Source: CAD feature listing. Evaluate the final solid. Frame: model axes, mm. A direction names the side the tool comes from. Round coordinates to 2 decimals unless told otherwise and drop trailing zeros. Write each loop counter-clockwise with the first axis right and the second up, starting at its lowest first coordinate (ties: lowest second). Pieces come first, ordered by that corner, then holes.
from build123d import *

# Parameters (mm, degrees)
F0_W     = 25.4
F0_H     = 25.4
F0_W_2   = 19.05
F0_H_2   = 19.05
F1_DEPTH = 1244.6


with BuildPart() as f1:
    # F0 (on Right) → F1 (new body)
    with BuildSketch(Plane.YZ):
        with Locations((12.7, 12.7)):
            Rectangle(F0_W, F0_H)
        with Locations((12.7, 12.7)):
            Rectangle(F0_W_2, F0_H_2, mode=Mode.SUBTRACT)
    extrude(amount=-F1_DEPTH)


solid = f1.part
1) Pull-direction query (Z, two-part tool) for faces 1 (the face through (-614, 13, 25.4)), 2 (the face through (-1244.6, 24, 13)), 3 (the face through (-614, 13, 22.225)); classes: released by +Z, released by -Z, zero draft, split by the parting line, or undercut.
Taken from the geometry:
face 1: released by +Z
face 2: zero draft
face 3: undercut
2) Contact query for a flat-ended pin moving along its axis: P1, Ø2, axis at x = -709.5, z = 21, coming from the -Y side. Output: stop coordinate, or through.
Taken from the geometry:
P1: stops at y = 0
3) Section query C-C on x = -1102.5. Return the cut outline in (y, z) (3 decimals), then the cut area to 3 significant figures.
Taken from the geometry:
outline: (0, 0) - (25.4, 0) - (25.4, 25.4) - (0, 25.4) - close; hole (3.175, 3.175) - (22.225, 3.175) - (22.225, 22.225) - (3.175, 22.225) - close
area: 282 mm2
4) Reachability of faces 4 (the face through (-614, 13, 3.175)), 5 (the face through (-614, 0, 13)) from +Z, -Z, +X, -X, +Y, -Y: full face, straight path, thin tool, end or side. Return the list, or none.
Taken from the geometry:
face 4: +X, -X
face 5: +Z, -Z, +X, -X, -Y
5) Section query A-A on z = 8. Return the cut outline in (x, y) (3 decimals), then the cut area to 3 significant figures.
Taken from the geometry:
outline: (-1244.6, 0) - (0, 0) - (0, 3.175) - (-1244.6, 3.175) - close; (-1244.6, 22.225) - (0, 22.225) - (0, 25.4) - (-1244.6, 25.4) - close
area: 7,900 mm2
6) Material intervals for line 1 (Z direction, x = -902, y = 19.5) (3 decimals), sorted ascending.
Taken from the geometry:
line 1: z = 0 to 3.175, 22.225 to 25.4
